```python
from build123d import *

# Parameters (mm, degrees)
BOSS_EXTRUDE1_DEPTH = 22
CUT_EXTRUDE1_DEPTH  = 4
CUT_EXTRUDE2_DEPTH  = 4
FILLET1_R           = 15
FILLET2_R           = 3


with BuildPart() as part:
    # Sketch1 → Boss-Extrude1 (new body)
    with BuildSketch(Plane.XY):
        Polygon((0, 0), (0, 15), (-3, 15), (-3, -3), (25, -3), (25, 0), align=None)
    extrude(amount=BOSS_EXTRUDE1_DEPTH)

    # Sketch2 → Cut-Extrude1 (cut, through all)
    with BuildSketch(Plane(origin=(0, 0, 0), x_dir=(1, 0, 0), z_dir=(0, 1, 0))):
        with BuildLine():
            Line((17, -1.75), (22, -1.75))
            ThreePointArc((22, -1.75), (23.75, -3.5), (22, -5.25))
            Line((22, -5.25), (17, -5.25))
            ThreePointArc((17, -5.25), (15.25, -3.5), (17, -1.75))
        make_face()
        with BuildLine():
            Line((17, -16.75), (22, -16.75))
            ThreePointArc((22, -16.75), (23.75, -18.5), (22, -20.25))
            Line((22, -20.25), (17, -20.25))
            ThreePointArc((17, -20.25), (15.25, -18.5), (17, -16.75))
        make_face()
    extrude(amount=-CUT_EXTRUDE1_DEPTH, mode=Mode.SUBTRACT)

    # Sketch3 → Cut-Extrude2 (cut, through all)
    with BuildSketch(Plane(origin=(0, 0, 0), x_dir=(0, 0, -1), z_dir=(1, 0, 0))):
        with BuildLine():
            Line((-10, 11.25), (-2, 11.25))
            ThreePointArc((-2, 11.25), (-0.75, 10), (-2, 8.75))
            Line((-2, 8.75), (-10, 8.75))
            ThreePointArc((-10, 8.75), (-11.25, 10), (-10, 11.25))
        make_face()
        with BuildLine():
            Line((-10, 5.25), (-2, 5.25))
            ThreePointArc((-2, 5.25), (-0.75, 4), (-2, 2.75))
            Line((-2, 2.75), (-10, 2.75))
            ThreePointArc((-10, 2.75), (-11.25, 4), (-10, 5.25))
        make_face()
    extrude(amount=-CUT_EXTRUDE2_DEPTH, mode=Mode.SUBTRACT)

    # Fillet1
    fillet1_edges = [part.edges().sort_by_distance(p)[0] for p in [
        (-1.5, 15, 22),
    ]]
    fillet(fillet1_edges, radius=FILLET1_R)

    # Fillet2
    fillet2_edges = [part.edges().sort_by_distance(p)[0] for p in [
        (25, -1.5, 22),
        (25, -1.5, 0),
        (-1.5, 15, 0),
    ]]
    fillet(fillet2_edges, radius=FILLET2_R)


solid = part.part
```
Design review of the part built by this model. Coordinates are the model's own, in mm. A direction names the side the tool comes from. Coordinates: 2 decimals unless noted, no trailing zeros. Loops run counter-clockwise (first coordinate to the right, second up) from the corner with the lowest first, then second, coordinate; pieces in that order, holes last. Notation, with made-up numbers: (24, 87) -> (41, 87) arc R17 cw to (41, 92) -> close; hole circle Ø8 at (20.5, 20). An arc over 180 degrees is marked (long way). Answer as a JSON object with one key per item and string values.
Q1. Tool access review of faces 1 (the flat face through (9, -1, 22)), 2 (the flat face through (13, 0, 11)), 3 (the flat face through (19, -1, 1.75)), 4 (the flat face through (-1, 5.25, 6)): name each direction out of +Z, -Z, +X, -X, +Y, -Y from which nothing blocks a thin tool from reaching the whole face with its end or side.
Answer block:
{"face 1": "+Z, +X, -X, +Y, -Y", "face 2": "+Z, -Z, +X, +Y", "face 3": "+Y, -Y", "face 4": "+X, -X"}
Q2. The part is to be moulded in two halves that separate along Y. For faces 5 (the cylindrical face through (-1.52, 10.49, 17.72)), 6 (the flat face through (11, -3, 11)), 7 (the cylindrical face through (15.25, -1.48, 18.54)), 8 (the cylindrical face through (-1.48, 10.03, 0.75)), say which applies: +Y half, -Y half, draft (parallel to the pull), parting line (faces both ways), or undercut.
Answer block:
{"face 5": "+Y half", "face 6": "-Y half", "face 7": "draft", "face 8": "undercut"}
Q3. Take a section at C-C on x = 19.25. Give the boundary of the cut face in (y, z), plus the area to 3 significant figures.
Answer block:
{"outline": "(-3, 0) -> (0, 0) -> (0, 1.75) -> (-3, 1.75) -> close; (-3, 5.25) -> (0, 5.25) -> (0, 16.75) -> (-3, 16.75) -> close; (-3, 20.25) -> (0, 20.25) -> (0, 22) -> (-3, 22) -> close", "area": "45.0 mm^2"}
Q4. Take a section at A-A on z = 3.5. Give the boundary of the cut face in (x, y).
Answer block:
{"outline": "(-3, -3) -> (15.25, -3) -> (15.25, 0) -> (0, 0) -> (0, 2.75) -> (-3, 2.75) -> close; (-3, 5.25) -> (0, 5.25) -> (0, 8.75) -> (-3, 8.75) -> close; (-3, 11.25) -> (0, 11.25) -> (0, 15) -> (-3, 15) -> close; (23.75, -3) -> (25, -3) -> (25, 0) -> (23.75, 0) -> close"}
Q5. Take a section at D-D on y = 4. Give the boundary of the cut face in (x, z), plus the area to 3 significant figures.
Answer block:
{"outline": "(-3, 0) -> (0, 0) -> (0, 0.75) -> (-3, 0.75) -> close; (-3, 11.25) -> (0, 11.25) -> (0, 21.46) -> (-3, 21.46) -> close", "area": "32.9 mm^2"}
Q6. Take a section at B-B on y = -1.5. Give the boundary of the cut face in (x, z).
Answer block:
{"outline": "(-3, 0) -> (22, 0) arc R3 ccw to (25, 3) -> (25, 19) arc R3 ccw to (22, 22) -> (-3, 22) -> close; hole (17, 1.75) -> (22, 1.75) arc R1.75 ccw to (22, 5.25) -> (17, 5.25) arc R1.75 ccw to start; hole (17, 16.75) -> (22, 16.75) arc R1.75 ccw to (22, 20.25) -> (17, 20.25) arc R1.75 ccw to start"}
Q7. Clearance check with flat-ended pins moving along their axes: pin 1 Ø6 at (y, z) = (8, 11.5) entering from +X; pin 2 Ø1.5 at (y, z) = (10, 3.5) entering from -X; pin 3 Ø2 at (x, y) = (0, 7.5) entering from +Z; pin 4 Ø6.5 at (x, z) = (18.5, 10.5) entering from +Y. State where each tip first meets the part, or that it passes through.
Answer block:
{"pin 1": "stops at x = 0", "pin 2": "passes through", "pin 3": "stops at z = 20.52", "pin 4": "stops at y = 0"}
Q8. To check wall thickness, follow L1, parallel to Y at x = 11.75, z = 12.25; L2, parallel to X at y = -2, z = 19. State the ranges of each line that lie inside material, in increasing order.
Answer block:
{"L1": "y = -3 to 0", "L2": "x = -3 to 15.32, 23.68 to 25"}
